from build123d import *

# Parameters (mm, degrees)
SKETCH1_W           = 126
SKETCH1_H           = 102
SKETCH1_R           = 12
SKETCH1_R_2         = 10
SKETCH1_W_2         = 3
SKETCH1_H_2         = 15
SKETCH1_W_3         = 15
SKETCH1_H_3         = 3
BOSS_EXTRUDE1_DEPTH = 3
SKETCH2_R           = 1.5
CUT_EXTRUDE1_DEPTH  = 3
CIRPATTERN1_COUNT   = 3
SKETCH3_R           = 1.5
CUT_EXTRUDE2_DEPTH  = 3
CIRPATTERN2_COUNT   = 4


with BuildPart() as part:
    # Sketch1 → Boss-Extrude1 (new body)
    with BuildSketch(Plane.XY):
        with Locations((12, 0)):
            Rectangle(SKETCH1_W, SKETCH1_H)
        with Locations((-24.15725, 0)):
            Circle(SKETCH1_R, mode=Mode.SUBTRACT)
        with Locations((24.15725, 0)):
            Circle(SKETCH1_R_2, mode=Mode.SUBTRACT)
        with Locations((-46.5, -35.5)):
            Rectangle(SKETCH1_W_2, SKETCH1_H_2, mode=Mode.SUBTRACT)
        with Locations((-46.5, 35.5)):
            Rectangle(SKETCH1_W_2, SKETCH1_H_2, mode=Mode.SUBTRACT)
        with Locations((70.5, -35.5)):
            Rectangle(SKETCH1_W_2, SKETCH1_H_2, mode=Mode.SUBTRACT)
        with Locations((70.5, 35.5)):
            Rectangle(SKETCH1_W_2, SKETCH1_H_2, mode=Mode.SUBTRACT)
        with Locations((-35.5, 46.5)):
            Rectangle(SKETCH1_W_3, SKETCH1_H_3, mode=Mode.SUBTRACT)
        with Locations((59.5, 46.5)):
            Rectangle(SKETCH1_W_3, SKETCH1_H_3, mode=Mode.SUBTRACT)
        with Locations((-35.5, -46.5)):
            Rectangle(SKETCH1_W_3, SKETCH1_H_3, mode=Mode.SUBTRACT)
        with Locations((59.5, -46.5)):
            Rectangle(SKETCH1_W_3, SKETCH1_H_3, mode=Mode.SUBTRACT)
    extrude(amount=BOSS_EXTRUDE1_DEPTH)

    # Sketch2 → Cut-Extrude1 (cut)
    with BuildSketch(Plane.XY.offset(3)):
        with Locations((24.15725, 15)):
            Circle(SKETCH2_R)
    cut_extrude1 = extrude(amount=-CUT_EXTRUDE1_DEPTH, mode=Mode.SUBTRACT)

    # CirPattern1: Cut-Extrude1 ×3 about axis
    cirpattern1_axis = Axis((24.15725, 0, 0), (0, 0, 1))
    for i in range(1, CIRPATTERN1_COUNT):
        add(cut_extrude1.rotate(cirpattern1_axis, i * 360 / CIRPATTERN1_COUNT), mode=Mode.SUBTRACT)

    # Sketch3 → Cut-Extrude2 (cut)
    with BuildSketch(Plane.XY.offset(3)):
        with Locations((-24.15725, 15)):
            Circle(SKETCH3_R)
    cut_extrude2 = extrude(amount=-CUT_EXTRUDE2_DEPTH, mode=Mode.SUBTRACT)

    # CirPattern2: Cut-Extrude2 ×4 about axis
    cirpattern2_axis = Axis((-24.15725, 0, 0), (0, 0, 1))
    for i in range(1, CIRPATTERN2_COUNT):
        add(cut_extrude2.rotate(cirpattern2_axis, i * 360 / CIRPATTERN2_COUNT), mode=Mode.SUBTRACT)


solid = part.part
For this review, take the finished solid that the model builds, in its own axes (mm). Give positions to 0.01 mm unless a question says otherwise; leave off trailing zeros. Loops run counter-clockwise (first coordinate to the right, second up) from the corner with the lowest first, then second, coordinate; pieces in that order, holes last. Notation, with made-up numbers: M -26,-25 L -5,-25 A21 cw -5,13 Z; hole C -25,-27.5 d6. An arc over 180 degrees is marked long. Put each result on its own line as item: value. Start each with the question number.
(1) For pin 1 (2.5 mm diameter, centred on x = -24.16, y = -15, fed in from -Z), flat-tipped, find the tip position at first contact; note if it passes through.
(2) Wall thickness on L1, parallel to Y at x = 65.5, z = 1.6; L2, parallel to Y at x = -24, z = 1.9; L3, parallel to X at y = 39, z = 0.2: over which ranges is each line inside the solid? List them lowest first.
(3) Add section C-C, the plane x = 55. Write out the cut boundary in (y, z).
(4) Add section A-A, the plane y = -15. Write out the cut boundary in (x, z).
(5) Add section B-B, the plane y = 32. Write out the cut boundary in (x, z), then the cut area to 3 significant figures.
(6) Add section D-D, the plane y = 0. Write out the cut boundary in (x, z), then the cut area to 3 significant figures.
Result:
1. pin 1: passes through
2. L1: y = -51 to -48, -45 to 45, 48 to 51
2. L2: y = -51 to -16.49, -13.51 to -12, 12 to 13.51, 16.49 to 51
2. L3: x = -51 to -48, -45 to 69, 72 to 75
3. outline: M -51,0 L -48,0 L -48,3 L -51,3 Z; M -45,0 L 45,0 L 45,3 L -45,3 Z; M 48,0 L 51,0 L 51,3 L 48,3 Z
4. outline: M -51,0 L -25.66,0 L -25.66,3 L -51,3 Z; M -22.66,0 L 75,0 L 75,3 L -22.66,3 Z
5. outline: M -51,0 L -48,0 L -48,3 L -51,3 Z; M -45,0 L 69,0 L 69,3 L -45,3 Z; M 72,0 L 75,0 L 75,3 L 72,3 Z
5. area: 360 mm^2
6. outline: M -51,0 L -40.66,0 L -40.66,3 L -51,3 Z; M -37.66,0 L -36.16,0 L -36.16,3 L -37.66,3 Z; M -12.16,0 L -10.66,0 L -10.66,3 L -12.16,3 Z; M -7.66,0 L 14.16,0 L 14.16,3 L -7.66,3 Z; M 34.16,0 L 75,0 L 75,3 L 34.16,3 Z
6. area: 228 mm^2
